Build history of the part. All positions in model axes, mm. Give positions to 0.01 mm unless a question says otherwise; leave off trailing zeros. Order: outer loops, then holes, each group sorted by start corner. A loop starts at its lowest first (then second) coordinate and runs counter-clockwise, first axis right, second up. Notation, with made-up numbers: (50.25, -13.75) - (83.25, -13.75) arc R23 cw to (83.25, 25.25) - close; hole circle Ø8 at (39, 37). An arc over 180 degrees is marked (long way). Write each question's results on one line, items separated by ' | '. Start each with the question number.
1) Drill centre lines: line 1 along X through (y, z) = (0, -14.5); line 2 along Z through (x, y) = (160.5, 0) (1 decimal); line 3 along Z through (x, y) = (291, -7). Where is each one in solid material? Low to high. Write a range as from..to.
2) Cut at A-A on z = 0. List the corners of the cut face in (x, y) (1 decimal).
3) Cut at B-B on x = 137.5. List the corners of the cut face in (y, z) (1 decimal), plus the area to 3 significant figures.
4) Drop flat-ended pins along their axis: pin 1 Ø4 at (x, y) = (246.5, 4) entering from -Z; pin 2 Ø4 at (x, z) = (252, 4.5) entering from +Y; pin 3 Ø1.5 at (x, z) = (56.5, -1.5) entering from -Y. Give the stop position or say it passes through.
from build123d import *

# Parameters (mm, degrees)
SKETCH1_R               = 16.7005
SKETCH1_R_2             = 13.335
BOSS_EXTRUDE1_DEPTH     = 355.6
SKETCH2_R               = 2.4257
CUT_EXTRUDE1_DEPTH      = 17.7005
CUT_EXTRUDE1_DEPTH_BACK = 17.7005


with BuildPart() as part:
    # Sketch1 → Boss-Extrude1 (new body)
    with BuildSketch(Plane(origin=(0, 0, 0), x_dir=(0, 0, -1), z_dir=(1, 0, 0))):
        Circle(SKETCH1_R)
        Circle(SKETCH1_R_2, mode=Mode.SUBTRACT)
    extrude(amount=BOSS_EXTRUDE1_DEPTH)

    # Sketch2 → Cut-Extrude1 (cut, two sides)
    with BuildSketch(Plane.XY) as cut_extrude1_sk:
        with Locations((209.55, 0)):
            Circle(SKETCH2_R)
        with Locations((260.35, 0)):
            Circle(SKETCH2_R)
    extrude(amount=CUT_EXTRUDE1_DEPTH, mode=Mode.SUBTRACT)
    extrude(cut_extrude1_sk.sketch, amount=-CUT_EXTRUDE1_DEPTH_BACK, mode=Mode.SUBTRACT)


solid = part.part
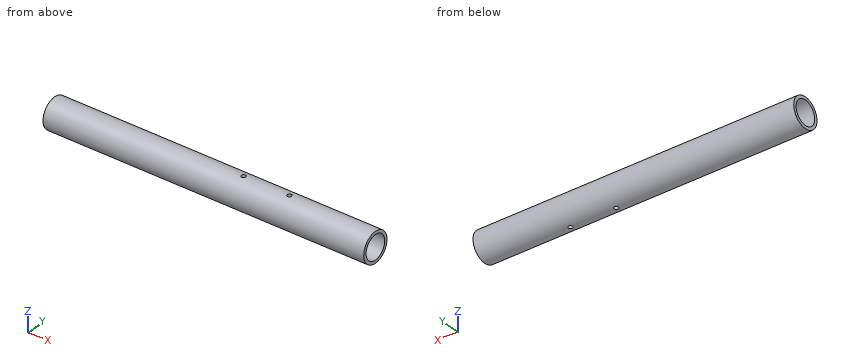
Results:
1) line 1: 0..207.12, 211.98..257.92, 262.78..355.6 | line 2: -16.7..-13.3, 13.3..16.7 | line 3: -15.16..-11.35, 11.35..15.16
2) outline: (0, -16.7) - (355.6, -16.7) - (355.6, -13.3) - (0, -13.3) - close; (0, 13.3) - (355.6, 13.3) - (355.6, 16.7) - (0, 16.7) - close
3) outline: circle Ø33.4 at (0, 0); hole circle Ø26.7 at (0, 0) | area: 318 mm^2
4) pin 1: z = -16.58 | pin 2: y = 16.51 | pin 3: y = -16.68
